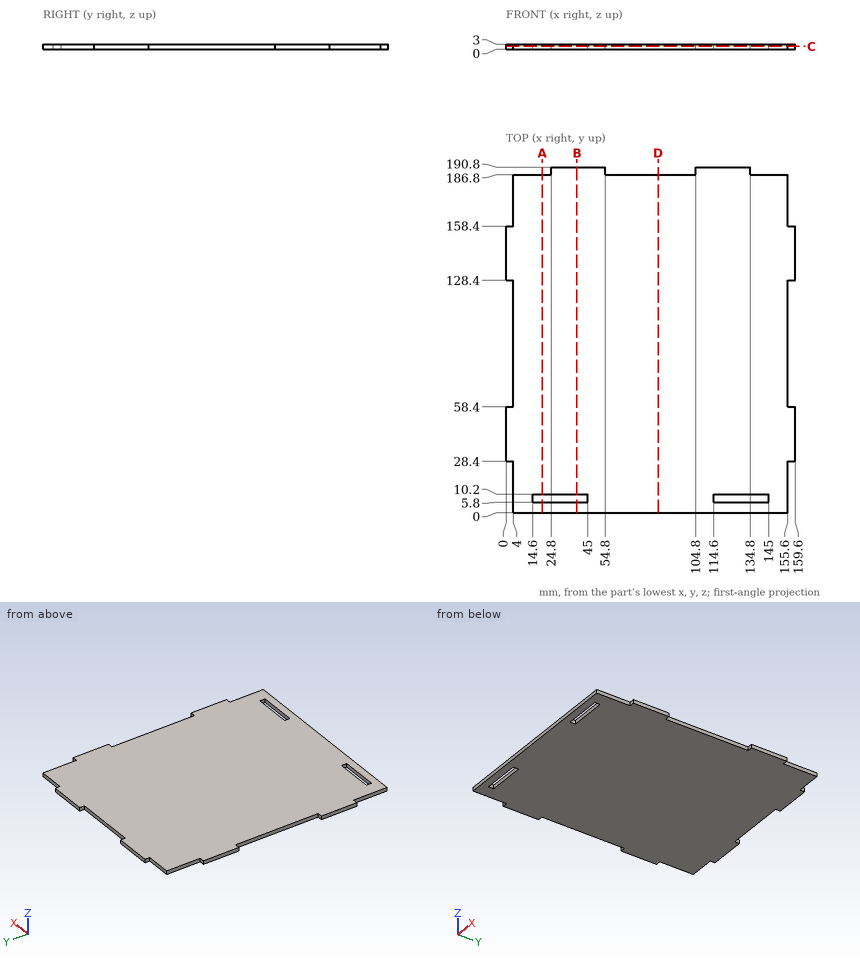
Geometry check sheet. Reference: drawing and pictorial views, mm from the part's lowest x, y, z. Give positions to 0.01 mm unless a question says otherwise; leave off trailing zeros. Order: outer loops, then holes, each group sorted by start corner. A loop starts at its lowest first (then second) coordinate and runs counter-clockwise, first axis right, second up. Notation, with made-up numbers: M 51,88.25 L 92,88.25 A4 cw 92,94.25 Z; hole C 25,30 d4. An arc over 180 degrees is marked long. Answer as a JSON object with one key per item and string values. Group by question number.
1) Cross-section at A-A (x = 20). Enter the section's corners in (y, z), then the cut area to 3 significant figures.
2) Scan lines: line 1 along Y through (x, z) = (28, 2.5); line 2 along X through (y, z) = (13.5, 1.95); line 3 along Y through (x, z) = (59, 2.3). Record each from-to range of solid material in increasing order. Write a range as [from, to].
3) Cross-section at D-D (x = 84). Enter the section's corners in (y, z).
4) Depth check by flat-ended pin: pin 1 Ø0.9 at (x, z) = (3, 1.5) entering from -Y; pin 2 Ø0.9 at (y, z) = (15.5, 1) entering from -X; pin 3 Ø1.5 at (x, z) = (72, 2.5) entering from -Y; pin 4 Ø1.5 at (y, z) = (80, 2) entering from +X. Enter the tip coordinate at first touch or a pass-through.
5) Cross-section at B-B (x = 39). Enter the section's corners in (y, z).
6) Cross-section at C-C (z = 1.75). Give the number of separate pieces and of enclosed holes in the cut face, then the cut area to 3 significant figures.
Result sheet:
{
 "1": {"outline": "M 0,0 L 5.8,0 L 5.8,3 L 0,3 Z; M 10.2,0 L 186.8,0 L 186.8,3 L 10.2,3 Z", "area": "547 mm2"},
 "2": {"line 1": "y = [0, 5.8], [10.2, 190.8]", "line 2": "x = [4, 155.6]", "line 3": "y = [0, 186.8]"},
 "3": {"outline": "M 0,0 L 186.8,0 L 186.8,3 L 0,3 Z"},
 "4": {"pin 1": "stops at y = 28.4", "pin 2": "stops at x = 4", "pin 3": "stops at y = 0", "pin 4": "stops at x = 155.6"},
 "5": {"outline": "M 0,0 L 5.8,0 L 5.8,3 L 0,3 Z; M 10.2,0 L 190.8,0 L 190.8,3 L 10.2,3 Z"},
 "6": {"separate pieces": "1", "enclosed holes": "2", "area": "28,800 mm2"}
}
